Input: part model. Units: mm. Frame: model coordinates. Face numbers are marked on the shaded views. A direction names the side the tool comes from. Give positions to 0.01 mm unless a question says otherwise; leave off trailing zeros. Loops run counter-clockwise (first coordinate to the right, second up) from the corner with the lowest first, then second, coordinate; pieces in that order, holes last. Notation, with made-up numbers: M 6,26 L 62,26 A28 ccw 62,47 Z; hole C -21,-8 d2. An arc over 180 degrees is marked long. Answer as a JSON object with one key per item and string values. Group by question number.
1) Section query A-A on y = 21. Return loops of the section in (x, z), plus the area to 3 significant figures.
2) Section query B-B on z = 40. Return loops of the section in (x, y).
3) Draft query along Z for the marked faces 3, 4 and 5. Return one class per face: +Z half, -Z half, draft (parallel to the pull), parting line (faces both ways), or undercut.
4) Section query D-D on z = 64. Return loops of the section in (x, y).
5) Ray query, L1, parallel to X at y = 46.5, z = 40; L2, parallel to X at y = 38.5, z = 70. Return the intervals inside material, ascending.
6) Access query for the marked faces 1 and 2. Directions: +Z, -Z, +X, -X, +Y, -Y. A direction counts if a zero-diameter tool reaches every point of the face in a straight line with its end or side. Return the directions, or none.
7) Section query C-C on x = 40. Return loops of the section in (y, z).
8) First-contact query: P1, Ø15, axis at x = 33.5, z = 42, coming from the +Y side; P2, Ø11, axis at x = 36.5, z = 34.5, coming from the -Y side. Flat tips, straight axial feed; report the tip coordinate or a pass-through.
from build123d import *

# Parameters (mm, degrees)
IZIM1_W                     = 80
IZIM1_H                     = 80
Y_KSEKLIK_EKSTR_ZYON1_DEPTH = 80
IZIM2_R                     = 15
KES_EKSTR_ZYON1_DEPTH       = 50
RADYUS1_R                   = 10
BO_ALTMA1_T                 = -3


with BuildPart() as part:
    # Çizim1 → Yükseklik-Ekstrüzyon1 (new body)
    with BuildSketch(Plane.XY):
        with Locations((40, 40)):
            Rectangle(IZIM1_W, IZIM1_H)
    extrude(amount=Y_KSEKLIK_EKSTR_ZYON1_DEPTH)

    # Çizim2 → Kes-Ekstrüzyon1 (cut)
    with BuildSketch(Plane(origin=(0, 80, 0), x_dir=(1, 0, 0), z_dir=(0, 1, 0))):
        with Locations(Location((40, -40, 0), (0, 0, 270))):
            Circle(IZIM2_R)
    extrude(amount=-KES_EKSTR_ZYON1_DEPTH, mode=Mode.SUBTRACT)

    # Radyus1
    radyus1_edges = [part.edges().sort_by_distance(p)[0] for p in [
        (80, 40, 80),
        (40, 80, 80),
        (0, 40, 80),
        (40, 80, 0),
        (80, 40, 0),
        (0, 40, 0),
        (0, 80, 40),
        (80, 80, 40),
    ]]
    fillet(radyus1_edges, radius=RADYUS1_R)

    # İç Boşaltma1
    bo_altma1_openings = [part.faces().sort_by_distance(p)[0] for p in [
        (40, 0, 40),
    ]]
    offset(amount=BO_ALTMA1_T, openings=bo_altma1_openings, kind=Kind.INTERSECTION)


solid = part.part
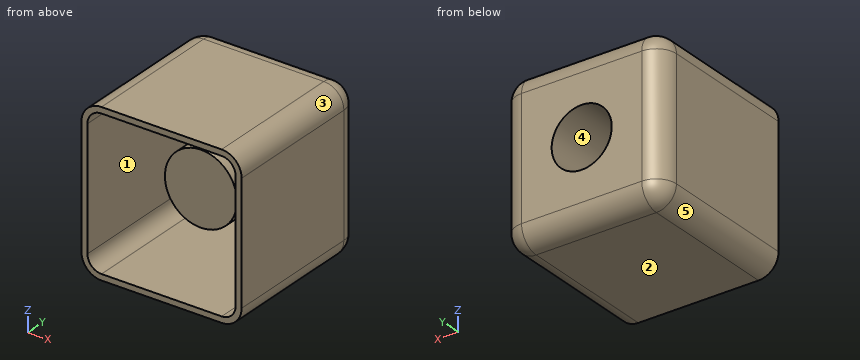
Output:
{
 "1": {"outline": "M 0,10 A10 ccw 10,0 L 70,0 A10 ccw 80,10 L 80,70 A10 ccw 70,80 L 10,80 A10 ccw 0,70 Z; hole M 3,10 A7 ccw 10,3 L 70,3 A7 ccw 77,10 L 77,70 A7 ccw 70,77 L 10,77 A7 ccw 3,70 Z", "area": "880 mm^2"},
 "2": {"outline": "M 0,0 L 3,0 L 3,70 A7 cw 10,77 L 22,77 L 22,27 L 58,27 L 58,77 L 70,77 A7 cw 77,70 L 77,0 L 80,0 L 80,70 A10 ccw 70,80 L 55,80 L 55,30 L 25,30 L 25,80 L 10,80 A10 ccw 0,70 Z"},
 "3": {"face 3": "+Z half", "face 4": "undercut", "face 5": "-Z half"},
 "4": {"outline": "M 0,0 L 3,0 L 3,70 A7 cw 10,77 L 70,77 A7 cw 77,70 L 77,0 L 80,0 L 80,70 A10 ccw 70,80 L 10,80 A10 ccw 0,70 Z"},
 "5": {"L1": "x = 0 to 3, 22 to 25, 55 to 58, 77 to 80", "L2": "x = 0 to 3, 77 to 80"},
 "6": {"face 1": "-Y", "face 2": "-Z, +X, -X, +Y, -Y"},
 "7": {"outline": "M 0,0 L 70,0 A10 ccw 80,10 L 80,25 L 30,25 L 30,55 L 80,55 L 80,70 A10 ccw 70,80 L 0,80 L 0,77 L 70,77 A7 cw 77,70 L 77,58 L 27,58 L 27,22 L 77,22 L 77,10 A7 cw 70,3 L 0,3 Z"},
 "8": {"P1": "stops at y = 30", "P2": "stops at y = 27"}
}
